Geometry check sheet. Reference: the model listing, model coordinates, mm. A direction names the side the tool comes from. Give positions to 0.01 mm unless a question says otherwise; leave off trailing zeros. Write each loop counter-clockwise with the first axis right and the second up, starting at its lowest first coordinate (ties: lowest second). Pieces come first, ordered by that corner, then holes. Notation, with made-up numbers: M 10.5,38.25 L 30.5,38.25 A20 ccw 30.5,55.25 Z; hole C 34.25,-2 d7. An arc over 180 degrees is marked long. One line per item, written item: value. Start each with the question number.
1. Cross-section at D-D on z = 3. Record the cut outline in (x, y), then the cut area to 3 significant figures.
2. Cross-section at A-A on x = 6.8. Record the cut outline in (y, z), then the cut area to 3 significant figures.
3. Tool access check on faces 4 (the face through (-33.8, 1.4, 9.7)), 5 (the face through (41, 0, 6)), 6 (the face through (22.46, 0.04, 9.55)), 7 (the face through (-29, 0, 4)), 8 (the face through (34, 0, 4)). Record the directions out of +Z, -Z, +X, -X, +Y, -Y that give a thin tool (end or side, any length) a straight path to the whole face; none if there is none.
4. Gauge pin test, flat ends, axial feed: pin 1 (3 mm diameter, centred on y = -1, z = 11.5, fed in from -X); pin 2 (1.3 mm diameter, centred on x = -33.8, z = 6, fed in from -Y); pin 3 (2 mm diameter, centred on y = 0, z = 10, fed in from -X); pin 4 (3 mm diameter, centred on y = 0, z = 10, fed in from +X). Record the tip position at first contact, or that the pin passes through.
5. Cross-section at B-B on y = 0. Record the cut outline in (x, z), then the cut area to 3 significant figures.
6. Scan lines: line 1 (Z direction, x = 6.8, y = 0.75); line 2 (X direction, y = 1.75, z = 3.25); line 3 (X direction, y = 1.5, z = 3). Record each from-to range of solid material in increasing order.
7. Release check for a two-part mould opening along Y. For faces 1 (the face through (7.99, -0.04, 3.38)), 2 (the face through (-21.8, 0, 10)), 3 (the face through (-22, 3, 6)) record: pulls with the +Y half, pulls with the -Y half, needs draft (parallel to the pull), parting line crosses it, or undercut.
8. Cross-section at C-C on z = 7.25. Record the cut outline in (x, y), then the cut area to 3 significant figures.
from build123d import *

# Parameters (mm, degrees)
F1_DEPTH  = 13
F2_W      = 10
F2_H      = 7
F3_DEPTH  = 6.001
F5_DEPTH  = 13.001
F6_R      = 1.25
F7_DEPTH  = 12
F8_R      = 1.25
F9_DEPTH  = 12
F10_R     = 1.25
F11_DEPTH = 6.001
F13_DEPTH = 6


with BuildPart() as f1:
    # F0 (on Top) → F1 (new body)
    with BuildSketch(Plane.XY):
        Polygon((38.8, 3), (-33.8, 3), (-33.8, -3), (-6, -3), (6, -3), (38.8, -3), align=None)
    extrude(amount=F1_DEPTH)

    # F2 (on face) → F3 (cut, through all)
    with BuildSketch(Plane(origin=(0, 3, 0), x_dir=(-1, 0, 0), z_dir=(0, 1, 0))):
        Polygon((-28.8, 7), (-28.8, 0), (-21.8, 0), align=None)
        with Locations((-33.8, 3.5)):
            Rectangle(F2_W, F2_H)
        Polygon((20.5147186258, 13), (-25.5147186258, 13), (-19.3147186258, 6), (14.3147186258, 6), align=None)
        Polygon((23.8, 7), (16.8, 0), (23.8, 0), align=None)
        with Locations((28.8, 3.5)):
            Rectangle(F2_W, F2_H)
    extrude(amount=-F3_DEPTH, mode=Mode.SUBTRACT)

    # F4 (on face) → F5 (cut, through all)
    with BuildSketch(Plane(origin=(0, 0, 0), x_dir=(1, 0, 0), z_dir=(0, 0, -1))):
        with BuildLine():
            Line((-6, -3), (6, -3))
            ThreePointArc((6, -3), (0, -0.7), (-6, -3))
        make_face()
    extrude(amount=-F5_DEPTH, mode=Mode.SUBTRACT)

    # F6 (on face) → F7 (cut)
    with BuildSketch(Plane.YZ.offset(38.8)):
        with Locations((0, 10)):
            Circle(F6_R)
    extrude(amount=-F7_DEPTH, mode=Mode.SUBTRACT)

    # F8 (on face) → F9 (cut)
    with BuildSketch(Plane(origin=(-33.8, 0, 0), x_dir=(0, -1, 0), z_dir=(-1, 0, 0))):
        with Locations((0, 10)):
            Circle(F8_R)
    extrude(amount=-F9_DEPTH, mode=Mode.SUBTRACT)

    # F10 (on face) → F11 (cut, through all)
    with BuildSketch(Plane.XZ.offset(3)):
        with Locations((-1.8, 3)):
            Circle(F10_R)
        with Locations((6.8, 3)):
            Circle(F10_R)
    extrude(amount=-F11_DEPTH, mode=Mode.SUBTRACT)

    # F12 (on face) → F13 (join)
    with BuildSketch(Plane.XZ.offset(3)):
        with BuildLine():
            Line((38.8, 6.5), (38.8, 7))
            Line((38.8, 7), (28.8, 7))
            Line((28.8, 7), (25.8, 4))
            Line((25.8, 4), (42.8, 4))
            Line((42.8, 4), (42.8, 6))
            Line((42.8, 6), (39.3, 6))
            ThreePointArc((39.3, 6), (38.4464466094, 5.6464466094), (38.8, 6.5))
        make_face()
        with BuildLine():
            Line((-37.8, 4), (-20.8, 4))
            Line((-20.8, 4), (-23.8, 7))
            Line((-23.8, 7), (-33.8, 7))
            Line((-33.8, 7), (-33.8, 6.5))
            ThreePointArc((-33.8, 6.5), (-33.4464466094, 5.6464466094), (-34.3, 6))
            Line((-34.3, 6), (-37.8, 6))
            Line((-37.8, 6), (-37.8, 4))
        make_face()
    extrude(amount=-F13_DEPTH)


solid = f1.part
Report:
1. outline: M -19.8,-3 L -3.05,-3 L -3.05,1.23 A8.98 cw -6,3 L -19.8,3 Z; M -0.55,-3 L 5.55,-3 L 5.55,2.62 A8.98 cw -0.55,0.72 Z; M 8.05,-3 L 24.8,-3 L 24.8,3 L 8.05,3 Z
1. area: 224 mm^2
2. outline: M -3,0 L 3,0 L 3,1.75 L -3,1.75 Z; M -3,4.25 L 3,4.25 L 3,6 L -3,6 Z
2. area: 21.0 mm^2
3. face 4: +Z, -X, +Y, -Y
3. face 5: +Z, +X, +Y, -Y
3. face 6: +Z, +Y, -Y
3. face 7: -Z, -X, +Y, -Y
3. face 8: -Z, +X, +Y, -Y
4. pin 1: stops at x = -33.8
4. pin 2: stops at y = -3
4. pin 3: stops at x = -21.8
4. pin 4: stops at x = 38.8
5. outline: M -37.8,4 L -20.8,4 L -16.8,0 L 21.8,0 L 25.8,4 L 42.8,4 L 42.8,6 L 39.3,6 A0.5 cw long 38.8,6.5 L 38.8,8.75 L 26.8,8.75 L 26.8,11.25 L 38.8,11.25 L 38.8,13 L 25.51,13 L 19.31,6 L -14.31,6 L -20.51,13 L -33.8,13 L -33.8,11.25 L -21.8,11.25 L -21.8,8.75 L -33.8,8.75 L -33.8,6.5 A0.5 cw long -34.3,6 L -37.8,6 Z; hole C -1.8,3 d2.5; hole C 6.8,3 d2.5
5. area: 490 mm^2
6. line 1: z = 0 to 1.75, 4.25 to 6
6. line 2: x = -20.05 to -4.21, 4.21 to 5.58, 8.02 to 25.05
6. line 3: x = -19.8 to -3.7, 3.7 to 5.55, 8.05 to 24.8
7. face 1: needs draft
7. face 2: undercut
7. face 3: pulls with the +Y half
8. outline: M -33.8,-3 L -15.42,-3 L -15.42,3 L -33.8,3 Z; M 20.42,-3 L 38.8,-3 L 38.8,3 L 20.42,3 Z
8. area: 221 mm^2
